from build123d import *

# Parameters (mm, degrees)
SKETCH_1_R          = 1.5
SKETCH_1_R_2        = 32.5
EXTRUDE_1_DEPTH     = 3
SKETCH_2_R          = 3.25
SKETCH_2_R_2        = 3.5
SKETCH_2_W          = 16
SKETCH_2_H          = 18
CUT_EXTRUDE_2_DEPTH = 10
FILLET_2_R          = 5
FILLET_3_R          = 2
CUT_EXTRUDE_START   = -10
SKETCH_3_R          = 1.5
SKETCH_3_R_2        = 32.5
CUT_EXTRUDE_3_DEPTH = 10
SKETCH_5_R          = 1.5
CUT_EXTRUDE_4_DEPTH = 10
SKETCH_6_R          = 1.5
CUT_EXTRUDE_5_DEPTH = 404.124050386
SKETCH_7_R          = 1.5
CUT_EXTRUDE_6_DEPTH = 404.124050386
SKETCH_8_W          = 45.011761124
SKETCH_8_H          = 18
CUT_EXTRUDE_7_DEPTH = 10
FILLET_4_R          = 3


with BuildPart() as part:
    # 草图1 → 凸台-拉伸1 (new body)
    with BuildSketch(Plane.XY):
        with BuildLine():
            Line((-10, 50), (-350, 50))
            ThreePointArc((-350, 50), (-400, 0), (-350, -50))
            Line((-350, -50), (-10, -50))
            ThreePointArc((-10, -50), (40, 0), (-10, 50))
        make_face()
        with Locations((-387.5, 0)):
            Circle(SKETCH_1_R, mode=Mode.SUBTRACT)
        with Locations((-378.726666617, 24.104535363)):
            Circle(SKETCH_1_R, mode=Mode.SUBTRACT)
        with Locations((-356.511806663, 36.930290738)):
            Circle(SKETCH_1_R, mode=Mode.SUBTRACT)
        with Locations((-331.25, 32.475952642)):
            Circle(SKETCH_1_R, mode=Mode.SUBTRACT)
        with Locations((-314.761526721, 12.825755375)):
            Circle(SKETCH_1_R, mode=Mode.SUBTRACT)
        with Locations((-314.761526721, -12.825755375)):
            Circle(SKETCH_1_R, mode=Mode.SUBTRACT)
        with Locations((-331.25, -32.475952642)):
            Circle(SKETCH_1_R, mode=Mode.SUBTRACT)
        with Locations((-356.511806663, -36.930290738)):
            Circle(SKETCH_1_R, mode=Mode.SUBTRACT)
        with Locations((-378.726666617, -24.104535363)):
            Circle(SKETCH_1_R, mode=Mode.SUBTRACT)
        with Locations((-350, 0)):
            Circle(SKETCH_1_R_2, mode=Mode.SUBTRACT)
        with Locations((-10, 0)):
            Circle(SKETCH_1_R_2, mode=Mode.SUBTRACT)
        with Locations((18.726666617, -24.104535363)):
            Circle(SKETCH_1_R, mode=Mode.SUBTRACT)
        with Locations((-3.488193337, -36.930290738)):
            Circle(SKETCH_1_R, mode=Mode.SUBTRACT)
        with Locations((-28.75, -32.475952642)):
            Circle(SKETCH_1_R, mode=Mode.SUBTRACT)
        with Locations((-45.238473279, -12.825755375)):
            Circle(SKETCH_1_R, mode=Mode.SUBTRACT)
        with Locations((-45.238473279, 12.825755375)):
            Circle(SKETCH_1_R, mode=Mode.SUBTRACT)
        with Locations((-28.75, 32.475952642)):
            Circle(SKETCH_1_R, mode=Mode.SUBTRACT)
        with Locations((-3.488193337, 36.930290738)):
            Circle(SKETCH_1_R, mode=Mode.SUBTRACT)
        with Locations((18.726666617, 24.104535363)):
            Circle(SKETCH_1_R, mode=Mode.SUBTRACT)
        with Locations((27.5, 0)):
            Circle(SKETCH_1_R, mode=Mode.SUBTRACT)
    extrude(amount=EXTRUDE_1_DEPTH)

    # 草图2 → 切除-拉伸2 (cut)
    with BuildSketch(Plane.XY.offset(3)):
        with Locations((-331.250850225, 32.476443505)):
            Circle(SKETCH_2_R)
        with Locations((-387.499999987, -0.000981748)):
            Circle(SKETCH_2_R_2)
        with Locations((-331.249149788, -32.475461757)):
            Circle(SKETCH_2_R)
        with Locations((-317.5, 0)):
            Rectangle(SKETCH_2_W, SKETCH_2_H)
    extrude(amount=-CUT_EXTRUDE_2_DEPTH, mode=Mode.SUBTRACT)

    # 圆角2
    fillet_2_edges = [part.edges().sort_by_distance(p)[0] for p in [
        (-318.771007061, -9, 1.5),
        (-318.771007061, 9, 1.5),
    ]]
    fillet(fillet_2_edges, radius=FILLET_2_R)

    # 圆角3
    fillet_3_edges = [part.edges().sort_by_distance(p)[0] for p in [
        (-309.5, 9, 1.5),
        (-309.5, -9, 1.5),
    ]]
    fillet(fillet_3_edges, radius=FILLET_3_R)

    # 草图3 → 切除-拉伸3 (cut)
    with BuildSketch(Plane.XY.offset(3).offset(CUT_EXTRUDE_START)):
        with BuildLine():
            Line((-280, -50), (-180, -50))
            Line((-180, -50), (-10, -50))
            ThreePointArc((-10, -50), (40, 0), (-10, 50))
            Line((-10, 50), (-280, 50))
            Line((-280, 50), (-280, -50))
        make_face()
        with Locations((-28.75, -32.475952642)):
            Circle(SKETCH_3_R, mode=Mode.SUBTRACT)
        with Locations((-3.488193337, -36.930290738)):
            Circle(SKETCH_3_R, mode=Mode.SUBTRACT)
        with Locations((18.726666617, -24.104535363)):
            Circle(SKETCH_3_R, mode=Mode.SUBTRACT)
        with Locations((-45.238473279, -12.825755375)):
            Circle(SKETCH_3_R, mode=Mode.SUBTRACT)
        with Locations((-45.238473279, 12.825755375)):
            Circle(SKETCH_3_R, mode=Mode.SUBTRACT)
        with Locations((-10, 0)):
            Circle(SKETCH_3_R_2, mode=Mode.SUBTRACT)
        with Locations((27.5, 0)):
            Circle(SKETCH_3_R, mode=Mode.SUBTRACT)
        with Locations((-28.75, 32.475952642)):
            Circle(SKETCH_3_R, mode=Mode.SUBTRACT)
        with Locations((18.726666617, 24.104535363)):
            Circle(SKETCH_3_R, mode=Mode.SUBTRACT)
        with Locations((-3.488193337, 36.930290738)):
            Circle(SKETCH_3_R, mode=Mode.SUBTRACT)
    extrude(amount=CUT_EXTRUDE_3_DEPTH, mode=Mode.SUBTRACT)

    # 草图5 → 切除-拉伸4 (cut)
    with BuildSketch(Plane.XY.offset(3)):
        with Locations((-396.25, 0)):
            Circle(SKETCH_5_R)
    extrude(amount=-CUT_EXTRUDE_4_DEPTH, mode=Mode.SUBTRACT)

    # 草图6 → 切除-拉伸5 (cut, through all)
    with BuildSketch(Plane.XY.offset(3)):
        with Locations((-396.25, 0)):
            Circle(SKETCH_6_R)
        with Locations((-373.125, 40.053674925)):
            Circle(SKETCH_6_R)
        with Locations((-326.875, 40.053674925)):
            Circle(SKETCH_6_R)
        with Locations((-303.75, 0)):
            Circle(SKETCH_6_R)
        with Locations((-326.875, -40.053674925)):
            Circle(SKETCH_6_R)
        with Locations((-373.125, -40.053674925)):
            Circle(SKETCH_6_R)
    extrude(amount=-CUT_EXTRUDE_5_DEPTH, mode=Mode.SUBTRACT)

    # 草图7 → 切除-拉伸6 (cut, through all)
    with BuildSketch(Plane.XY.offset(3)):
        with Locations((-309.987078995, 40.056872182)):
            Circle(SKETCH_7_R)
        with Locations((-289.987080036, 40.050420343)):
            Circle(SKETCH_7_R)
        with Locations((-309.998951455, -40.050946012)):
            Circle(SKETCH_7_R)
        with Locations((-289.998951462, -40.050422413)):
            Circle(SKETCH_7_R)
    extrude(amount=-CUT_EXTRUDE_6_DEPTH, mode=Mode.SUBTRACT)

    # 草图8 → 切除-拉伸7 (cut)
    with BuildSketch(Plane.XY.offset(3)):
        with Locations((-290.849795651, 0)):
            Rectangle(SKETCH_8_W, SKETCH_8_H)
    extrude(amount=-CUT_EXTRUDE_7_DEPTH, mode=Mode.SUBTRACT)

    # 圆角4
    fillet_4_edges = [part.edges().sort_by_distance(p)[0] for p in [
        (-280, -9, 1.5),
        (-280, 9, 1.5),
    ]]
    fillet(fillet_4_edges, radius=FILLET_4_R)


solid = part.part
Work out the finished part from the listing and answer in its coordinate system (mm). A direction names the side the tool comes from. Give positions to 0.01 mm unless a question says otherwise; leave off trailing zeros. Order: outer loops, then holes, each group sorted by start corner. A loop starts at its lowest first (then second) coordinate and runs counter-clockwise, first axis right, second up. Notation, with made-up numbers: (23.25, -26.5) -> (36.25, -26.5) arc R22 cw to (36.25, 0.5) -> close; hole circle Ø8 at (27.25, -4). An arc over 180 degrees is marked (long way). One line per item, written item: value.
Item 1: Find section B-B, the plane z = 0.7. State how many separate pieces and enclosed holes the cut face has, plus the area to 3 significant figures.
Answer sheet:
separate pieces: 1
enclosed holes: 18
area: 6,710 mm²
Item 2: A tool of negligible diameter and unlimited length cuts with its end or side. For faces 1 (the flat face through (-280, -31, 1)), 2 (the cylindrical face through (-280.9, -9.86, 1.48)), 3 (the cylindrical face through (-318.045, 9.88, 1.479)), from which of +Z, -Z, +X, -X, +Y, -Y can it reach the whole face along a straight path? Write none if from no direction.
Answer sheet:
face 1: +Z, -Z, +X, +Y, -Y
face 2: +Z, -Z, +X
face 3: +Z, -Z
Item 3: Find section C-C, the plane x = -396.25. Give the vertices of the cut face in (y, z), plus the area to 3 significant figures.
Answer sheet:
outline: (-19, 0) -> (-1.5, 0) -> (-1.5, 3) -> (-19, 3) -> close; (1.5, 0) -> (19, 0) -> (19, 3) -> (1.5, 3) -> close
area: 105 mm²
Item 4: Determine the mould class of faces 4 (the flat face through (-314, -10, 0)), 5 (the cylindrical face through (-371.694, -39.603, 1.521)), 6 (the cylindrical face through (-280.86, 9.9, 1.48)), 7 (the cylindrical face through (-291.5, -40, 1.5)) for opening direction X: released by +X, released by -X, zero draft, split by the parting line, or undercut.
Answer sheet:
face 4: zero draft
face 5: undercut
face 6: released by +X
face 7: undercut
Item 5: Straight lines are drawn through the part: probe 1 along Y at (x, z) = (-378, 0.45); probe 2 along X at (y, z) = (-24, 1.25); probe 3 along Y at (x, z) = (-309, 0.7). For each, find the intervals that lie inside material, in ascending order.
Answer sheet:
probe 1: -41.42 to -25.42, -22.79 to -16.5, 16.5 to 22.79, 25.42 to 41.42
probe 2: -393.86 to -380.22, -377.23 to -371.91, -328.09 to -280
probe 3: -50 to -41.17, -38.93 to -9, 9 to 38.93, 41.19 to 50
Item 6: Find section A-A, the plane x = -348. Give the vertices of the cut face in (y, z).
Answer sheet:
outline: (-50, 0) -> (-32.44, 0) -> (-32.44, 3) -> (-50, 3) -> close; (32.44, 0) -> (50, 0) -> (50, 3) -> (32.44, 3) -> close
Item 7: Flat-ended cylindrical pins translate along their axes: P1, Ø1, axis at x = -387.5, z = 2, coming from the -Y side; P2, Ø1.5, axis at x = -375.5, z = 1.5, coming from the +Y side; P3, Ø5, axis at x = -314.76, y = 12.83, coming from the +Z side; P4, Ø1.5, axis at x = -373.5, z = 2, coming from the +Y side. Find the tip coordinate at first contact, or state that the pin passes through.
Answer sheet:
P1: y = -33.63
P2: y = 43.44
P3: z = 3
P4: y = 44.52
